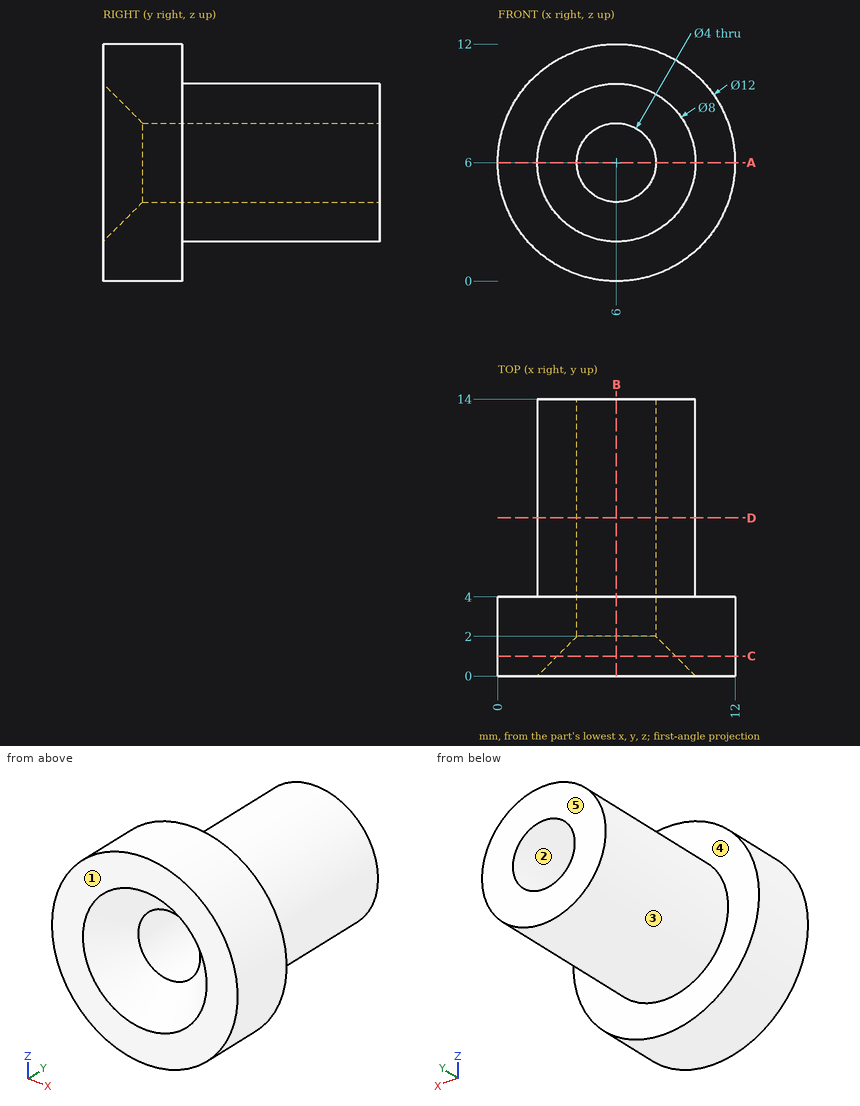
Here's the drawing with two shaded views (mm, measured from the low corner). I have some questions. A direction names the side the tool comes from. Coordinates: 2 decimals unless noted, no trailing zeros. Loops run counter-clockwise (first coordinate to the right, second up) from the corner with the lowest first, then second, coordinate; pieces in that order, holes last. Notation, with made-up numbers: (30.25, 84.25) -> (78.25, 84.25) arc R18 cw to (78.25, 109.25) -> close; hole circle Ø11 at (43.25, 5.25). An arc over 180 degrees is marked (long way). Answer in a Markdown table with one row per item.
(1) Will these pins go through, and if not, where does the flat tip stop? pin 1 Ø6 at (x, y) = (3, 6) entering from +Z; pin 2 Ø5 at (y, z) = (10, 9) entering from +X; pin 3 Ø2 at (x, y) = (7.5, 7.5) entering from -Z; pin 4 Ø5 at (x, z) = (6, 6) entering from +Y.
Results found:
| item | result |
|---|---|
| pin 1 | stops at z = 11.95 |
| pin 2 | stops at x = 9.97 |
| pin 3 | stops at z = 2.03 |
| pin 4 | stops at y = 14 |
(2) Imagine slicing it at D-D (y = 8). List the corners of the cut face in (x, z) for me, plus the area to 3 significant figures.
Results found:
| item | result |
|---|---|
| outline | circle Ø8 at (6, 6); hole circle Ø4 at (6, 6) |
| area | 37.7 mm^2 |
(3) If I drill on probe 1 along Z at (x, y) = (6, 6.25); probe 2 along Z at (x, y) = (6, 3), over which ranges is the centre line in solid material (lowest first)?
Results found:
| item | result |
|---|---|
| probe 1 | z = 2 to 4, 8 to 10 |
| probe 2 | z = 0 to 4, 8 to 12 |
(4) Imagine slicing it at B-B (x = 6). List the corners of the cut face in (y, z) for me.
Results found:
| item | result |
|---|---|
| outline | (0, 0) -> (4, 0) -> (4, 2) -> (14, 2) -> (14, 4) -> (2, 4) -> (0, 2) -> close; (0, 10) -> (2, 8) -> (14, 8) -> (14, 10) -> (4, 10) -> (4, 12) -> (0, 12) -> close |
(5) Imagine slicing it at C-C (y = 1). List the corners of the cut face in (x, z) for me, plus the area to 3 significant figures.
Results found:
| item | result |
|---|---|
| outline | circle Ø12 at (6, 6); hole circle Ø6 at (6, 6) |
| area | 84.8 mm^2 |
(6) Imagine slicing it at A-A (z = 6). List the corners of the cut face in (x, y) for me.
Results found:
| item | result |
|---|---|
| outline | (0, 0) -> (2, 0) -> (4, 2) -> (4, 14) -> (2, 14) -> (2, 4) -> (0, 4) -> close; (8, 2) -> (10, 0) -> (12, 0) -> (12, 4) -> (10, 4) -> (10, 14) -> (8, 14) -> close |
(7) For the marked faces 4 and 5, which set-ups out of +Z, -Z, +X, -X, +Y, -Y let a thin tool reach every point of the face, with its end or its side?
Results found:
| item | result |
|---|---|
| face 4 | +Y |
| face 5 | +Z, -Z, +X, -X, +Y |
(8) Thinking about a two-plate mould opening in X: for the marked faces 1, 2 and 3, which applies, released by +X, released by -X, zero draft, split by the parting line, or undercut?
Results found:
| item | result |
|---|---|
| face 1 | zero draft |
| face 2 | undercut |
| face 3 | split by the parting line |
